from build123d import *


with BuildPart() as f1:
    # F0 (on Right) → F1 (revolve)
    with BuildSketch(Plane.YZ):
        Polygon((0, 60.9), (0, 18.9), (59.7, 18.9), (59.7, 23.45), (80.6, 23.45), (80.6, 40), (55.5, 40), (55.5, 60.9), (52.8, 60.9), (49.45, 51.9), (47.45, 51.9), (44.1, 60.9), (39, 60.9), (35.65, 51.9), (33.65, 51.9), (30.3, 60.9), (25.2, 60.9), (21.85, 51.9), (19.85, 51.9), (16.5, 60.9), (11.4, 60.9), (8.05, 51.9), (6.05, 51.9), (2.7, 60.9), align=None)
    revolve(axis=Axis((0, 40.3, 0), (0, 1, 0)))


solid = f1.part
Could you check a few things on this model? Use its own coordinates, in mm. A direction names the side the tool comes from. Coordinates: 2 decimals unless noted, no trailing zeros. Loops run counter-clockwise (first coordinate to the right, second up) from the corner with the lowest first, then second, coordinate; pieces in that order, holes last.
1. Imagine slicing it at A-A (y = 62.5). Please give me the cut outline in (x, z), and give its area (3 significant figures).
2. We'd pull the mould along Y, two halves only. Please class faces 1 (the face through (-59.452, 41.514, -13.202)), 2 (the face through (-17, 80.6, -17)), 3 (the face through (-51.22, 19.64, -11.37)), 4 (the face through (15.721, 35.813, 49.92)): released by +Y, released by -Y, zero draft, split by the parting line, or undercut.
3. For P1, Ø3, axis at x = -20, y = 30.5, coming from the -Z side; P2, Ø23.5, axis at x = 3, z = -10, coming from the +Y side; P3, Ø5, axis at x = 42, y = 37.5, coming from the +Z side, each with a flat end and sliding along its axis, tell me the tip position at first contact or that it passes through.
4. Imagine slicing it at B-B (y = 27). Please give me the cut outline in (x, z).
5. I need wall thicknesses on L1, parallel to Z at x = -0.5, y = 14; L2, parallel to X at y = 16, z = 0; L3, parallel to X at y = 66.5, z = 0. Which ranges of each line are inside material? Lowest first, please.
6. For faces 5 (the face through (5.677, 30.268, 18.027)), 6 (the face through (-19.88, 7.04, 47.94)), 7 (the face through (-39.05, 67.87, -8.67)), which set-ups out of +Z, -Z, +X, -X, +Y, -Y let a thin tool reach every point of the face, with its end or its side?
Computed values:
1. outline: circle Ø80 at (0, 0); hole circle Ø46.9 at (0, 0)
1. area: 3,300 mm2
2. face 1: zero draft
2. face 2: released by +Y
2. face 3: undercut
2. face 4: undercut
3. P1: stops at z = -58.02
3. P2: stops at y = 59.7
3. P3: stops at z = 45.92
4. outline: circle Ø121.8 at (0, 0); hole circle Ø37.8 at (0, 0)
5. L1: z = -60.9 to -18.89, 18.89 to 60.9
5. L2: x = -60.9 to -18.9, 18.9 to 60.9
5. L3: x = -40 to -23.45, 23.45 to 40
6. face 5: +Y, -Y
6. face 6: none
6. face 7: +Y
